Geometry: final body of the model. Coordinates: model frame, mm. Coordinates: 2 decimals unless noted, no trailing zeros. Order: outer loops, then holes, each group sorted by start corner. A loop starts at its lowest first (then second) coordinate and runs counter-clockwise, first axis right, second up. Notation, with made-up numbers: M 66,9 L 109,9 A31 cw 109,41 Z; hole C 5,-8.75 d10. An arc over 180 degrees is marked long. Write item = value, one per line.
from build123d import *

# Parameters (mm, degrees)
F1_DEPTH = 7.62
F3_D     = 25.4
F5_D     = 25.4


with BuildPart() as f1:
    # F0 (on Top) → F1 (new body)
    with BuildSketch(Plane.XY):
        with BuildLine():
            ThreePointArc((41.275, 76.2), (0, 34.925), (-41.275, 76.2))
            ThreePointArc((-41.275, 76.2), (-100.895704, 100.895704), (-76.2, 41.275))
            ThreePointArc((-76.2, 41.275), (-34.925, 0), (-76.2, -41.275))
            ThreePointArc((-76.2, -41.275), (-100.895704, -100.895704), (-41.275, -76.2))
            ThreePointArc((-41.275, -76.2), (0, -34.925), (41.275, -76.2))
            ThreePointArc((41.275, -76.2), (100.895704, -100.895704), (76.2, -41.275))
            ThreePointArc((76.2, -41.275), (34.925, 0), (76.2, 41.275))
            ThreePointArc((76.2, 41.275), (100.895704, 100.895704), (41.275, 76.2))
        make_face()
    extrude(amount=F1_DEPTH)

    # F3 (through all)
    with Locations(Plane(origin=(0, 0, 0), x_dir=(1, 0, 0), z_dir=(0, 0, -1))):
        with Locations((-76.199986, 76.200023)):
            Hole(F3_D / 2)

    # F5 (through all)
    with Locations(Plane(origin=(0, 0, 0), x_dir=(1, 0, 0), z_dir=(0, 0, -1))):
        with Locations((-76.199934, -76.200038), (76.200068, -76.200001), (76.200128, 76.199986)):
            Hole(F5_D / 2)


solid = f1.part
1) Section A-A, the plane x = 81.5. Return loops of the section in (y, z), and give its area (3 significant figures).
Numbers:
outline = M -110.72,0 L -87.74,0 L -87.74,7.62 L -110.72,7.62 Z; M -64.66,0 L -41.68,0 L -41.68,7.62 L -64.66,7.62 Z; M 41.68,0 L 64.66,0 L 64.66,7.62 L 41.68,7.62 Z; M 87.74,0 L 110.72,0 L 110.72,7.62 L 87.74,7.62 Z
area = 700 mm²
2) Section B-B, the plane z = 3.25. Return loops of the section in (x, y) (3 decimals).
Numbers:
outline = M -76.2,-41.275 A34.925 ccw long -41.275,-76.2 A41.275 cw 41.275,-76.2 A34.925 ccw long 76.2,-41.275 A41.275 cw 76.2,41.275 A34.925 ccw long 41.275,76.2 A41.275 cw -41.275,76.2 A34.925 ccw long -76.2,41.275 A41.275 cw Z; hole C -76.2,-76.2 d25.4; hole C -76.2,76.2 d25.4; hole C 76.2,-76.2 d25.4; hole C 76.2,76.2 d25.4
3) Line query: L1, parallel to X at y = -76.5, z = 1.75; L2, parallel to X at y = -75, z = 7; L3, parallel to Y at x = 67, z = 6.25. Output: solid intervals per line, ascending.
Numbers:
L1 = -111.12 to -88.9, -63.5 to -41.28, 41.28 to 63.5, 88.9 to 111.12
L2 = -111.1 to -88.84, -63.56 to -41.26, 41.26 to 63.56, 88.84 to 111.1
L3 = -109.89 to -84.95, -67.45 to -40.24, 40.24 to 67.45, 84.95 to 109.89
4) Mould query, pull axis Y, two halves, no side actions, for faces 1 (the face through (-0.908, -34.935, 3.757)), 2 (the face through (0.908, 34.935, 3.757)), 3 (the face through (-2, 2, 0)), 4 (the face through (77.853, -88.792, 3.863)). Classes: pulls with the +Y half, pulls with the -Y half, needs draft (parallel to the pull), parting line crosses it, or undercut.
Numbers:
face_1 = pulls with the -Y half
face_2 = pulls with the +Y half
face_3 = needs draft
face_4 = undercut
5) Pin query (flat end, axial travel): pin 1 (2 mm diameter, centred on x = -27, z = 1, fed in from +Y); pin 2 (15 mm diameter, centred on x = -76.2, y = -76.2, fed in from -Z); pin 3 (2 mm diameter, centred on x = -4.5, z = 7, fed in from +Y); pin 4 (1.5 mm diameter, centred on x = -15, z = 4, fed in from -Y). Return the tip coordinate at first contact, or that it passes through.
Numbers:
pin_1 = 45.87
pin_2 = through
pin_3 = 35.29
pin_4 = -38.05
6) Section C-C, the plane y = 0. Return loops of the section in (x, z) (3 decimals).
Numbers:
outline = M -34.925,0 L 34.925,0 L 34.925,7.62 L -34.925,7.62 Z
